```python
from build123d import *

# Parameters (mm, degrees)
ESQUISSE1_W             = 160
ESQUISSE1_H             = 310
ESQUISSE1_R             = 2.5
ESQUISSE1_R_2           = 2.75
ESQUISSE1_R_3           = 2.25
BOSS_EXTRU_1_DEPTH      = 12
ESQUISSE2_R             = 4.5
ENL_V_MAT_EXTRU_1_DEPTH = 5
ENL_V_MAT_EXTRU_2_REACH = 351.062
ESQUISSE3_R             = 2.25
ENL_V_MAT_EXTRU_3_REACH = 351.062
ESQUISSE4_R             = 5
ESQUISSE5_R             = 8.5
ENL_V_MAT_EXTRU_4_DEPTH = 6


with BuildPart() as part:
    # Esquisse1 → Boss.-Extru.1 (new body)
    with BuildSketch(Plane.XY):
        with Locations((80, 155)):
            Rectangle(ESQUISSE1_W, ESQUISSE1_H)
        with Locations((97.5, 15)):
            Circle(ESQUISSE1_R, mode=Mode.SUBTRACT)
        with Locations((127.5, 15)):
            Circle(ESQUISSE1_R, mode=Mode.SUBTRACT)
        with Locations((97.5, 47)):
            Circle(ESQUISSE1_R, mode=Mode.SUBTRACT)
        with Locations((127.5, 47)):
            Circle(ESQUISSE1_R, mode=Mode.SUBTRACT)
        with Locations(Location((62.5, 47, 0), (0, 0, 180))):
            Circle(ESQUISSE1_R, mode=Mode.SUBTRACT)
        with Locations(Location((32.5, 47, 0), (0, 0, 180))):
            Circle(ESQUISSE1_R, mode=Mode.SUBTRACT)
        with Locations(Location((32.5, 15, 0), (0, 0, 180))):
            Circle(ESQUISSE1_R, mode=Mode.SUBTRACT)
        with Locations(Location((62.5, 15, 0), (0, 0, 180))):
            Circle(ESQUISSE1_R, mode=Mode.SUBTRACT)
        with Locations((57, 30)):
            Circle(ESQUISSE1_R_2, mode=Mode.SUBTRACT)
        with Locations(Location((103, 30, 0), (0, 0, 180))):
            Circle(ESQUISSE1_R_2, mode=Mode.SUBTRACT)
        with Locations((57, 279)):
            Circle(ESQUISSE1_R_2, mode=Mode.SUBTRACT)
        with Locations(Location((103, 279, 0), (0, 0, 180))):
            Circle(ESQUISSE1_R_2, mode=Mode.SUBTRACT)
        with Locations((15, 216.85)):
            Circle(ESQUISSE1_R_3, mode=Mode.SUBTRACT)
        with Locations((80, 216.85)):
            Circle(ESQUISSE1_R_3, mode=Mode.SUBTRACT)
        with Locations((145, 216.85)):
            Circle(ESQUISSE1_R_3, mode=Mode.SUBTRACT)
    extrude(amount=BOSS_EXTRU_1_DEPTH)

    # Esquisse2 → Enlèv. mat.-Extru.1 (cut)
    with BuildSketch(Plane.XY.offset(12)):
        with Locations((32.5, 47)):
            Circle(ESQUISSE2_R)
        with Locations((32.5, 15)):
            Circle(ESQUISSE2_R)
        with Locations((62.5, 15)):
            Circle(ESQUISSE2_R)
        with Locations((62.5, 47)):
            Circle(ESQUISSE2_R)
        with Locations(Location((127.5, 15, 0), (0, 0, 180))):
            Circle(ESQUISSE2_R)
        with Locations(Location((97.5, 15, 0), (0, 0, 180))):
            Circle(ESQUISSE2_R)
        with Locations(Location((97.5, 47, 0), (0, 0, 180))):
            Circle(ESQUISSE2_R)
        with Locations(Location((127.5, 47, 0), (0, 0, 180))):
            Circle(ESQUISSE2_R)
        with Locations((15, 216.85)):
            Circle(ESQUISSE2_R)
        with Locations((80, 216.85)):
            Circle(ESQUISSE2_R)
        with Locations((145, 216.85)):
            Circle(ESQUISSE2_R)
    extrude(amount=-ENL_V_MAT_EXTRU_1_DEPTH, mode=Mode.SUBTRACT)

    # Esquisse3 → Enlèv. mat.-Extru.2 (cut, up to next)
    with BuildSketch(Plane.XY.offset(12), mode=Mode.PRIVATE) as enl_v_mat_extru_2_sk1:
        with Locations((155, 25)):
            Circle(ESQUISSE3_R)
    enl_v_mat_extru_2_tool1 = extrude(enl_v_mat_extru_2_sk1.sketch, amount=-ENL_V_MAT_EXTRU_2_REACH, mode=Mode.PRIVATE) & part.part
    # Esquisse3 → Enlèv. mat.-Extru.2 (cut, up to next)
    with BuildSketch(Plane.XY.offset(12), mode=Mode.PRIVATE) as enl_v_mat_extru_2_sk2:
        with Locations((125, 25)):
            Circle(ESQUISSE3_R)
    enl_v_mat_extru_2_tool2 = extrude(enl_v_mat_extru_2_sk2.sketch, amount=-ENL_V_MAT_EXTRU_2_REACH, mode=Mode.PRIVATE) & part.part
    # Esquisse3 → Enlèv. mat.-Extru.2 (cut, up to next)
    with BuildSketch(Plane.XY.offset(12), mode=Mode.PRIVATE) as enl_v_mat_extru_2_sk3:
        with Locations((125, 115)):
            Circle(ESQUISSE3_R)
    enl_v_mat_extru_2_tool3 = extrude(enl_v_mat_extru_2_sk3.sketch, amount=-ENL_V_MAT_EXTRU_2_REACH, mode=Mode.PRIVATE) & part.part
    # Esquisse3 → Enlèv. mat.-Extru.2 (cut, up to next)
    with BuildSketch(Plane.XY.offset(12), mode=Mode.PRIVATE) as enl_v_mat_extru_2_sk4:
        with Locations((125, 205)):
            Circle(ESQUISSE3_R)
    enl_v_mat_extru_2_tool4 = extrude(enl_v_mat_extru_2_sk4.sketch, amount=-ENL_V_MAT_EXTRU_2_REACH, mode=Mode.PRIVATE) & part.part
    # Esquisse3 → Enlèv. mat.-Extru.2 (cut, up to next)
    with BuildSketch(Plane.XY.offset(12), mode=Mode.PRIVATE) as enl_v_mat_extru_2_sk5:
        with Locations((125, 295)):
            Circle(ESQUISSE3_R)
    enl_v_mat_extru_2_tool5 = extrude(enl_v_mat_extru_2_sk5.sketch, amount=-ENL_V_MAT_EXTRU_2_REACH, mode=Mode.PRIVATE) & part.part
    # Esquisse3 → Enlèv. mat.-Extru.2 (cut, up to next)
    with BuildSketch(Plane.XY.offset(12), mode=Mode.PRIVATE) as enl_v_mat_extru_2_sk6:
        with Locations((155, 115)):
            Circle(ESQUISSE3_R)
    enl_v_mat_extru_2_tool6 = extrude(enl_v_mat_extru_2_sk6.sketch, amount=-ENL_V_MAT_EXTRU_2_REACH, mode=Mode.PRIVATE) & part.part
    # Esquisse3 → Enlèv. mat.-Extru.2 (cut, up to next)
    with BuildSketch(Plane.XY.offset(12), mode=Mode.PRIVATE) as enl_v_mat_extru_2_sk7:
        with Locations((155, 205)):
            Circle(ESQUISSE3_R)
    enl_v_mat_extru_2_tool7 = extrude(enl_v_mat_extru_2_sk7.sketch, amount=-ENL_V_MAT_EXTRU_2_REACH, mode=Mode.PRIVATE) & part.part
    # Esquisse3 → Enlèv. mat.-Extru.2 (cut, up to next)
    with BuildSketch(Plane.XY.offset(12), mode=Mode.PRIVATE) as enl_v_mat_extru_2_sk8:
        with Locations((155, 295)):
            Circle(ESQUISSE3_R)
    enl_v_mat_extru_2_tool8 = extrude(enl_v_mat_extru_2_sk8.sketch, amount=-ENL_V_MAT_EXTRU_2_REACH, mode=Mode.PRIVATE) & part.part
    # Esquisse3 → Enlèv. mat.-Extru.2 (cut, up to next)
    with BuildSketch(Plane.XY.offset(12), mode=Mode.PRIVATE) as enl_v_mat_extru_2_sk9:
        with Locations(Location((5, 295, 0), (0, 0, 180))):
            Circle(ESQUISSE3_R)
    enl_v_mat_extru_2_tool9 = extrude(enl_v_mat_extru_2_sk9.sketch, amount=-ENL_V_MAT_EXTRU_2_REACH, mode=Mode.PRIVATE) & part.part
    # Esquisse3 → Enlèv. mat.-Extru.2 (cut, up to next)
    with BuildSketch(Plane.XY.offset(12), mode=Mode.PRIVATE) as enl_v_mat_extru_2_sk10:
        with Locations(Location((35, 295, 0), (0, 0, 180))):
            Circle(ESQUISSE3_R)
    enl_v_mat_extru_2_tool10 = extrude(enl_v_mat_extru_2_sk10.sketch, amount=-ENL_V_MAT_EXTRU_2_REACH, mode=Mode.PRIVATE) & part.part
    # Esquisse3 → Enlèv. mat.-Extru.2 (cut, up to next)
    with BuildSketch(Plane.XY.offset(12), mode=Mode.PRIVATE) as enl_v_mat_extru_2_sk11:
        with Locations(Location((5, 205, 0), (0, 0, 180))):
            Circle(ESQUISSE3_R)
    enl_v_mat_extru_2_tool11 = extrude(enl_v_mat_extru_2_sk11.sketch, amount=-ENL_V_MAT_EXTRU_2_REACH, mode=Mode.PRIVATE) & part.part
    # Esquisse3 → Enlèv. mat.-Extru.2 (cut, up to next)
    with BuildSketch(Plane.XY.offset(12), mode=Mode.PRIVATE) as enl_v_mat_extru_2_sk12:
        with Locations(Location((35, 205, 0), (0, 0, 180))):
            Circle(ESQUISSE3_R)
    enl_v_mat_extru_2_tool12 = extrude(enl_v_mat_extru_2_sk12.sketch, amount=-ENL_V_MAT_EXTRU_2_REACH, mode=Mode.PRIVATE) & part.part
    # Esquisse3 → Enlèv. mat.-Extru.2 (cut, up to next)
    with BuildSketch(Plane.XY.offset(12), mode=Mode.PRIVATE) as enl_v_mat_extru_2_sk13:
        with Locations(Location((35, 115, 0), (0, 0, 180))):
            Circle(ESQUISSE3_R)
    enl_v_mat_extru_2_tool13 = extrude(enl_v_mat_extru_2_sk13.sketch, amount=-ENL_V_MAT_EXTRU_2_REACH, mode=Mode.PRIVATE) & part.part
    # Esquisse3 → Enlèv. mat.-Extru.2 (cut, up to next)
    with BuildSketch(Plane.XY.offset(12), mode=Mode.PRIVATE) as enl_v_mat_extru_2_sk14:
        with Locations(Location((5, 115, 0), (0, 0, 180))):
            Circle(ESQUISSE3_R)
    enl_v_mat_extru_2_tool14 = extrude(enl_v_mat_extru_2_sk14.sketch, amount=-ENL_V_MAT_EXTRU_2_REACH, mode=Mode.PRIVATE) & part.part
    # Esquisse3 → Enlèv. mat.-Extru.2 (cut, up to next)
    with BuildSketch(Plane.XY.offset(12), mode=Mode.PRIVATE) as enl_v_mat_extru_2_sk15:
        with Locations(Location((35, 25, 0), (0, 0, 180))):
            Circle(ESQUISSE3_R)
    enl_v_mat_extru_2_tool15 = extrude(enl_v_mat_extru_2_sk15.sketch, amount=-ENL_V_MAT_EXTRU_2_REACH, mode=Mode.PRIVATE) & part.part
    # Esquisse3 → Enlèv. mat.-Extru.2 (cut, up to next)
    with BuildSketch(Plane.XY.offset(12), mode=Mode.PRIVATE) as enl_v_mat_extru_2_sk16:
        with Locations(Location((5, 25, 0), (0, 0, 180))):
            Circle(ESQUISSE3_R)
    enl_v_mat_extru_2_tool16 = extrude(enl_v_mat_extru_2_sk16.sketch, amount=-ENL_V_MAT_EXTRU_2_REACH, mode=Mode.PRIVATE) & part.part
    add(enl_v_mat_extru_2_tool1.solids().sort_by_distance((155, 25, 12))[0], mode=Mode.SUBTRACT)
    add(enl_v_mat_extru_2_tool2.solids().sort_by_distance((125, 25, 12))[0], mode=Mode.SUBTRACT)
    add(enl_v_mat_extru_2_tool3.solids().sort_by_distance((125, 115, 12))[0], mode=Mode.SUBTRACT)
    add(enl_v_mat_extru_2_tool4.solids().sort_by_distance((125, 205, 12))[0], mode=Mode.SUBTRACT)
    add(enl_v_mat_extru_2_tool5.solids().sort_by_distance((125, 295, 12))[0], mode=Mode.SUBTRACT)
    add(enl_v_mat_extru_2_tool6.solids().sort_by_distance((155, 115, 12))[0], mode=Mode.SUBTRACT)
    add(enl_v_mat_extru_2_tool7.solids().sort_by_distance((155, 205, 12))[0], mode=Mode.SUBTRACT)
    add(enl_v_mat_extru_2_tool8.solids().sort_by_distance((155, 295, 12))[0], mode=Mode.SUBTRACT)
    add(enl_v_mat_extru_2_tool9.solids().sort_by_distance((5, 295, 12))[0], mode=Mode.SUBTRACT)
    add(enl_v_mat_extru_2_tool10.solids().sort_by_distance((35, 295, 12))[0], mode=Mode.SUBTRACT)
    add(enl_v_mat_extru_2_tool11.solids().sort_by_distance((5, 205, 12))[0], mode=Mode.SUBTRACT)
    add(enl_v_mat_extru_2_tool12.solids().sort_by_distance((35, 205, 12))[0], mode=Mode.SUBTRACT)
    add(enl_v_mat_extru_2_tool13.solids().sort_by_distance((35, 115, 12))[0], mode=Mode.SUBTRACT)
    add(enl_v_mat_extru_2_tool14.solids().sort_by_distance((5, 115, 12))[0], mode=Mode.SUBTRACT)
    add(enl_v_mat_extru_2_tool15.solids().sort_by_distance((35, 25, 12))[0], mode=Mode.SUBTRACT)
    add(enl_v_mat_extru_2_tool16.solids().sort_by_distance((5, 25, 12))[0], mode=Mode.SUBTRACT)

    # Esquisse4 → Enlèv. mat.-Extru.3 (cut, up to next)
    with BuildSketch(Plane.XY.offset(12), mode=Mode.PRIVATE) as enl_v_mat_extru_3_sk1:
        with Locations((55, 73)):
            Circle(ESQUISSE4_R)
    enl_v_mat_extru_3_tool1 = extrude(enl_v_mat_extru_3_sk1.sketch, amount=-ENL_V_MAT_EXTRU_3_REACH, mode=Mode.PRIVATE) & part.part
    # Esquisse4 → Enlèv. mat.-Extru.3 (cut, up to next)
    with BuildSketch(Plane.XY.offset(12), mode=Mode.PRIVATE) as enl_v_mat_extru_3_sk2:
        with Locations((75, 73)):
            Circle(ESQUISSE4_R)
    enl_v_mat_extru_3_tool2 = extrude(enl_v_mat_extru_3_sk2.sketch, amount=-ENL_V_MAT_EXTRU_3_REACH, mode=Mode.PRIVATE) & part.part
    # Esquisse4 → Enlèv. mat.-Extru.3 (cut, up to next)
    with BuildSketch(Plane.XY.offset(12), mode=Mode.PRIVATE) as enl_v_mat_extru_3_sk3:
        with Locations((75, 123)):
            Circle(ESQUISSE4_R)
    enl_v_mat_extru_3_tool3 = extrude(enl_v_mat_extru_3_sk3.sketch, amount=-ENL_V_MAT_EXTRU_3_REACH, mode=Mode.PRIVATE) & part.part
    # Esquisse4 → Enlèv. mat.-Extru.3 (cut, up to next)
    with BuildSketch(Plane.XY.offset(12), mode=Mode.PRIVATE) as enl_v_mat_extru_3_sk4:
        with Locations((55, 123)):
            Circle(ESQUISSE4_R)
    enl_v_mat_extru_3_tool4 = extrude(enl_v_mat_extru_3_sk4.sketch, amount=-ENL_V_MAT_EXTRU_3_REACH, mode=Mode.PRIVATE) & part.part
    add(enl_v_mat_extru_3_tool1.solids().sort_by_distance((55, 73, 12))[0], mode=Mode.SUBTRACT)
    add(enl_v_mat_extru_3_tool2.solids().sort_by_distance((75, 73, 12))[0], mode=Mode.SUBTRACT)
    add(enl_v_mat_extru_3_tool3.solids().sort_by_distance((75, 123, 12))[0], mode=Mode.SUBTRACT)
    add(enl_v_mat_extru_3_tool4.solids().sort_by_distance((55, 123, 12))[0], mode=Mode.SUBTRACT)

    # Esquisse5 → Enlèv. mat.-Extru.4 (cut)
    with BuildSketch(Plane.XY.offset(12)):
        with Locations((55, 123)):
            Circle(ESQUISSE5_R)
        with Locations((75, 123)):
            Circle(ESQUISSE5_R)
        with Locations((75, 73)):
            Circle(ESQUISSE5_R)
        with Locations((55, 73)):
            Circle(ESQUISSE5_R)
    extrude(amount=-ENL_V_MAT_EXTRU_4_DEPTH, mode=Mode.SUBTRACT)


solid = part.part
```
Geometry check sheet. Reference: the model listing, model coordinates, mm. A direction names the side the tool comes from. Round coordinates to 2 decimals unless told otherwise and drop trailing zeros. Loops run counter-clockwise (first coordinate to the right, second up) from the corner with the lowest first, then second, coordinate; pieces in that order, holes last. Notation, with made-up numbers: (67, -23) - (114, -23) arc R12 cw to (114, -8) - close; hole circle Ø10 at (83.25, 6). An arc over 180 degrees is marked (long way). Use a Markdown table: item, result.
Q1. Cross-section at A-A on y = 73. Record the cut outline in (x, z).
Solutions:
| item | result |
|---|---|
| outline | (0, 0) - (50, 0) - (50, 6) - (46.5, 6) - (46.5, 12) - (0, 12) - close; (60, 0) - (70, 0) - (70, 6) - (66.5, 6) - (66.5, 12) - (63.5, 12) - (63.5, 6) - (60, 6) - close; (80, 0) - (160, 0) - (160, 12) - (83.5, 12) - (83.5, 6) - (80, 6) - close |
Q2. Material ranges on line 1 (Y direction, x = 32.5, z = 10.3); line 2 (X direction, y = 216.85, z = 2.75); line 3 (Y direction, x = 103, z = 7.25), recorded low to high.
Solutions:
| item | result |
|---|---|
| line 1 | y = 0 to 10.5, 19.5 to 42.5, 51.5 to 310 |
| line 2 | x = 0 to 12.75, 17.25 to 77.75, 82.25 to 142.75, 147.25 to 160 |
| line 3 | y = 0 to 27.25, 32.75 to 276.25, 281.75 to 310 |
Q3. Access from +Z, -Z, +X, -X, +Y, -Y to the whole of each face (thin tool, end or side, straight path). Record for faces 1 (the flat face through (17, 215, 7)), 2 (the cylindrical face through (51, 126, 3)).
Solutions:
| item | result |
|---|---|
| face 1 | +Z |
| face 2 | +Z, -Z |
Q4. Go/stop test with flat-tipped pins: P1, Ø4.5, axis at x = 33, y = 15.5, coming from the +Z side; P2, Ø13.5, axis at x = 75, y = 72, coming from the +Z side. Record where each tip stops, or that it passes through.
Solutions:
| item | result |
|---|---|
| P1 | stops at z = 7 |
| P2 | stops at z = 6 |
Q5. Cross-section at B-B on z = 3. State how many separate pieces and enclosed holes the cut face has, plus the area to 3 significant figures.
Solutions:
| item | result |
|---|---|
| separate pieces | 1 |
| enclosed holes | 35 |
| area | 48,700 mm2 |
Q6. Draft check along Y on faces 3 (the flat face through (160, 153, 6)), 4 (the cylindrical face through (79.619, 71.085, 3.042)), 5 (the flat face through (79, 0, 6)). Enter one of: released by +Y, released by -Y, zero draft, split by the parting line, or undercut.
Solutions:
| item | result |
|---|---|
| face 3 | zero draft |
| face 4 | undercut |
| face 5 | released by -Y |
